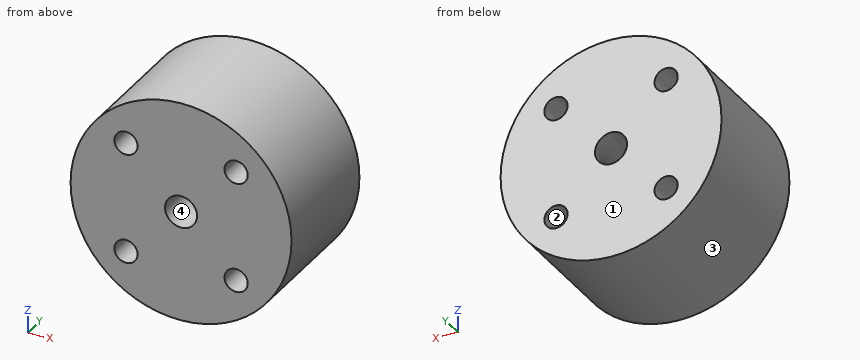
Autodesk Inventor part; units mm, degrees
ref_plane "YZ Plane" through (0, 0, 0) normal (1, 0, 0) x (0, 1, 0)
ref_plane "XZ Plane" through (0, 0, 0) normal (0, 1, 0) x (-1, 0, 0)
ref_plane "XY Plane" through (0, 0, 0) normal (0, 0, 1) x (1, 0, 0)
sketch "Sketch1" plane through (0, 0, 0) normal (0, 1, 0) x (-1, 0, 0)
  circle A0 centre (0, 0) radius 12.065
  line L0 (0, 0) -> (6.0168, -6.0168)
  line L1 (0, 0) -> (8.509, 0) construction
  circle A1 centre (6.0168, -6.0168) radius 1.27
  circle A2 centre (6.0168, 6.0168) radius 1.27
  circle A3 centre (-6.0168, 6.0168) radius 1.27
  circle A4 centre (-6.0168, -6.0168) radius 1.27
  dimension "d0" = 24.13
  dimension "d1" = 45
  dimension "d2" = 8.509
  dimension "d3" = 2.54
  dimension "d6" = 360
extrude "Extrusion1" add sketch "Sketch1" along normal blind 13.97
sketch "Sketch6" plane through (0, 13.97, 0) normal (0, 1, 0) x (1, 0, 0)
  circle A0 centre (0, 0) radius 1.75
  dimension "d32" = 3.5
extrude "Extrusion3" cut sketch "Sketch6" against normal through all
sketch "Sketch3" plane through (0, 13.97, 0) normal (0, 1, 0) x (1, 0, 0)
  circle A0 centre (0, 0) radius 1.75
  dimension "d14" = 3.5
sketch "Sketch7" plane through (0, 0, 0) normal (0, 0, 1) x (1, 0, 0)
  arc A0 (0, 13.97) -> (7.9375, 6.0325) centre (7.9375, 13.97) ccw
  line L0 (7.9375, 6.0325) -> (8.1915, 6.0325)
  point P0 (0, 0)
  dimension "d27" = 7.9375
  dimension "d28" = 7.9375
  dimension "d31" = 0.254
sweep "Sweep2" cut profiles "Sketch3" path "Sketch7"
properties part number "1PieceAttachment" material "ABS Plastic"
Design review of the part built by this model. Coordinates are the model's own, in mm. Face numbers are marked on the shaded views. Give positions to 0.01 mm unless a question says otherwise; leave off trailing zeros. Order: outer loops, then holes, each group sorted by start corner. A loop starts at its lowest first (then second) coordinate and runs counter-clockwise, first axis right, second up. Notation, with made-up numbers: (38.25, 72.25) - (80.25, 72.25) arc R28 cw to (80.25, 108.25) - close; hole circle Ø6 at (-35, 61.5). An arc over 180 degrees is marked (long way). Use a Markdown table: item, result. Add a question column.
(1) Clearance check with flat-ended pins moving along their axes: P1, Ø2, axis at x = 8.5, y = 2.5, coming from the +Z side; P2, Ø5.5, axis at x = 0, z = 0, coming from the +Y side. State where each tip first meets the part, or that it passes through.
(2) Add section B-B on z = -0.75. Give the boundary of the cut face in (x, y).
(3) Wall thickness on probe 1 along Z at (x, y) = (5.5, 4.5); probe 2 along Z at (x, y) = (-5, 7.25); probe 3 along Z at (x, y) = (0, 6.5) (3 decimals): over which ranges is each line inside the solid? List them lowest first. Write a range as [from, to].
(4) Add section C-C on x = 5.75. Give the number of separate pieces and of enclosed holes in the cut face, then the cut area to 3 significant figures.
(5) Mouldability with a two-part tool opening along X and no side actions: class the marked faces 1, 2, 3 and 4 as +X half, -X half, draft (parallel to the pull), parting line (faces both ways), or undercut.
(6) Add section A-A on z = 6.5. Give the boundary of the cut face in (x, y), then the cut area to 3 significant figures.
Report:
| question | item | result |
|---|---|---|
| 1 | P1 | stops at z = 9.45 |
| 1 | P2 | stops at y = 13.97 |
| 2 | outline | (-12.04, 0) - (-1.58, 0) - (-1.58, 13.97) - (-12.04, 13.97) - close; (1.58, 0) - (12.04, 0) - (12.04, 13.97) - (1.58, 13.97) arc R6.36 ccw to (7.94, 7.61) - (8.19, 7.61) - (8.19, 4.45) - (7.94, 4.45) arc R9.52 cw to (1.58, 6.88) - close |
| 3 | probe 1 | z = [-10.74, -7.18], [-4.86, 4.86], [7.18, 10.74] |
| 3 | probe 2 | z = [-10.98, -6.78], [-5.26, 5.26], [6.78, 10.98] |
| 3 | probe 3 | z = [-12.065, -1.75], [1.75, 12.065] |
| 4 | separate pieces | 3 |
| 4 | enclosed holes | 1 |
| 4 | area | 217 mm² |
| 5 | face 1 | draft |
| 5 | face 2 | undercut |
| 5 | face 3 | parting line |
| 5 | face 4 | undercut |
| 6 | outline | (-10.16, 0) - (-7.19, 0) - (-7.19, 13.97) - (-10.16, 13.97) - close; (-4.84, 0) - (4.84, 0) - (4.84, 13.97) - (-4.84, 13.97) - close; (7.19, 0) - (10.16, 0) - (10.16, 13.97) - (7.19, 13.97) - close |
| 6 | area | 218 mm² |
